Autodesk Inventor part; units mm, degrees
ref_plane "YZ Plane" through (0, 0, 0) normal (1, 0, 0) x (0, 1, 0)
ref_plane "XZ Plane" through (0, 0, 0) normal (0, 1, 0) x (-1, 0, 0)
ref_plane "XY Plane" through (0, 0, 0) normal (0, 0, 1) x (1, 0, 0)
sketch "Boceto1" plane through (0, 0, 0) normal (0, 0, 1) x (1, 0, 0)
  line L0 (567.5, -510) -> (-567.5, -510)
  line L1 (-567.5, -510) -> (-567.5, 510)
  line L2 (-567.5, 510) -> (567.5, 510)
  line L3 (567.5, 510) -> (567.5, -510)
  line L4 (567.5, -510) -> (-567.5, 510) construction
  line L5 (-567.5, -510) -> (567.5, 510) construction
  line L6 (605.6, 548.1) -> (-605.6, 548.1)
  line L7 (-605.6, 548.1) -> (-605.6, -548.1)
  line L8 (-605.6, -548.1) -> (605.6, -548.1)
  line L9 (605.6, -548.1) -> (605.6, 548.1)
  point P0 (0, 0)
  dimension "d0" = 1135
  dimension "d1" = 1020
  dimension "d2" = 38.1
extrude "Extrusión1" add sketch "Boceto1" along normal blind 38.1
fillet "Empalme1" radius 2 8 edges at (605.6, 548.1, 19.05) (605.6, -548.1, 19.05) (-605.6, 548.1, 19.05) (-605.6, -548.1, 19.05) (-567.5, -510, 19.05) (-567.5, 510, 19.05) (567.5, 510, 19.05) (567.5, -510, 19.05)
fillet "Empalme2" radius 2 24 edges at (-605.0142, 547.5142, 38.1) (-605.6, 0, 38.1) (-605.0142, -547.5142, 38.1) (0, -548.1, 38.1) (605.0142, -547.5142, 38.1) (605.6, 0, 38.1) (605.0142, 547.5142, 38.1) (0, 548.1, 38.1) (567.5, 0, 38.1) (0, -510, 38.1) (-567.5, 0, 38.1) (0, 510, 38.1) (-605.0142, 547.5142, 0) (-605.6, 0, 0) (-605.0142, -547.5142, 0) (0, -548.1, 0) (605.0142, -547.5142, 0) (605.6, 0, 0) (605.0142, 547.5142, 0) (0, 548.1, 0) (567.5, 0, 0) (0, -510, 0) (-567.5, 0, 0) (0, 510, 0)
sketch "Boceto2" plane through (0, 0, 0) normal (0, 0, -1) x (-1, 0, 0)
  line L0 (-603.6, 546.1) -> (-603.6, -546.1)
  line L1 (-603.6, 546.1) -> (-543.6, 546.1)
  line L2 (603.6, 546.1) -> (-603.6, 546.1)
  line L3 (-603.6, 548.1) -> (603.6, 548.1)
  line L4 (-543.6, 548.1) -> (-547.6, 548.1)
  line L5 (-543.6, 548.1) -> (-543.6, 544.1)
  line L6 (-543.6, 544.1) -> (-521.6, 544.1)
  line L7 (-521.6, 544.1) -> (-521.6, 548.1)
  line L8 (-521.6, 548.1) -> (-543.6, 548.1)
  line L9 (-543.6, 548.1) -> (-543.6, 544.1)
  line L10 (0, 548.1) -> (0, -512)
  line L11 (565.5, -512) -> (-565.5, -512)
  line L12 (-565.5, 0) -> (567.5, 0)
  line L13 (567.5, -508) -> (567.5, 508)
  line L14 (-603.6, -548.1) -> (603.6, -548.1)
  line L15 (-543.6, -548.1) -> (-543.6, -544.1)
  line L16 (-543.6, -544.1) -> (-521.6, -544.1)
  line L17 (-521.6, -544.1) -> (-521.6, -548.1)
  line L18 (543.6, 548.1) -> (543.6, 544.1)
  line L19 (543.6, 544.1) -> (521.6, 544.1)
  line L20 (521.6, 544.1) -> (521.6, 548.1)
  line L21 (521.6, 548.1) -> (543.6, 548.1)
  line L22 (543.6, -544.1) -> (521.6, -544.1)
  line L23 (521.6, -544.1) -> (521.6, -548.1)
  line L24 (603.6, -548.1) -> (-603.6, -548.1)
  line L25 (543.6, -548.1) -> (543.6, -544.1)
  point P0 (0, 0)
  point P1 (543.6, 546.1)
  dimension "d7" = 60
  dimension "d8" = 4
  dimension "d9" = 4
  dimension "d10" = 22
extrude "Extrusión2" add sketch "Boceto2" along normal blind 40 contours L18 L19 L20 L2 | L2 L20 L3 L18 | L7 L6 L5 L2 | L2 L5 L3 L7 | L15 L16 L17 L14 | L23 L22 L25 L14
fillet "Empalme3" radius 10 8 edges at (543.6, -546.1, -40) (521.6, -546.1, -40) (543.6, 546.1, -40) (521.6, 546.1, -40) (-521.6, 546.1, -40) (-543.6, 546.1, -40) (-543.6, -546.1, -40) (-521.6, -546.1, -40)
sketch "Boceto3" plane through (521.6, -548.1, 0) normal (0, -1, 0) x (1, 0, 0)
  line L0 (22, 0) -> (0, 0)
  line L1 (0, 0) -> (22, 0)
  line L2 (22, 0) -> (22, -40)
  line L3 (22, -40) -> (0, -40)
  line L4 (0, -40) -> (0, 0)
  circle A0 centre (11, -29) radius 11
  circle A1 centre (11, -29) radius 5
  point P0 (-521.6, 0)
  dimension "d14" = 10
extrude "Extrusión3" cut sketch "Boceto3" against normal blind 20000 contours A1
sketch "Boceto4" plane through (-543.6, -548.1, 0) normal (0, -1, 0) x (1, 0, 0)
  line L0 (0, 0) -> (0, -30)
  line L1 (0, 0) -> (22, 0)
  line L2 (22, 0) -> (22, -40)
  line L3 (22, -40) -> (0, -40)
  line L4 (0, -40) -> (0, 0)
  circle A0 centre (11, -29) radius 11
  circle A1 centre (11, -29) radius 5
  point P0 (543.6, 0)
  dimension "d17" = 10
extrude "Extrusión4" cut sketch "Boceto4" against normal blind 20000 contours A1
sketch "Boceto5" plane through (0, 0, 38.1) normal (0, 0, 1) x (1, 0, 0)
  line L0 (-565.5, 510) -> (565.5, 510)
  line L1 (565.5, -510) -> (-565.5, -510)
  point P0 (0, 0)
  dimension "d20" = 1020
sketch "Boceto6" plane through (0, 0, 38.1) normal (0, 0, 1) x (1, 0, 0)
  line L0 (565.5, -510) -> (-565.5, -510)
  line L1 (543.6, -548.1) -> (521.6, -548.1)
  line L2 (565.5, -510) -> (527.4, -510)
  line L3 (527.4, -510) -> (527.4, -548.1)
  line L4 (527.4, -548.1) -> (565.5, -548.1)
  line L5 (565.5, -548.1) -> (565.5, -510)
  line L6 (555.5, -538.1) -> (537.4, -538.1)
  line L7 (537.4, -538.1) -> (537.4, -520)
  line L8 (537.4, -520) -> (555.5, -520)
  line L9 (555.5, -520) -> (555.5, -538.1)
  circle A0 centre (555.5, -538.1) radius 2.5
  circle A1 centre (555.5, -520) radius 2.5
  circle A2 centre (537.4, -538.1) radius 2.5
  circle A3 centre (537.4, -520) radius 2.5
  line L10 (0, 0) -> (0, -570.6664)
  line L11 (0, 0) -> (796.3032, 0)
  line L12 (-565.5, -510) -> (-527.4, -510)
  line L13 (-527.4, -510) -> (-527.4, -548.1)
  line L14 (-527.4, -548.1) -> (-565.5, -548.1)
  line L15 (-565.5, -548.1) -> (-565.5, -510)
  circle A4 centre (-555.5, -538.1) radius 2.5
  circle A5 centre (-555.5, -520) radius 2.5
  circle A6 centre (-537.4, -538.1) radius 2.5
  circle A7 centre (-537.4, -520) radius 2.5
  line L16 (565.5, 510) -> (-565.5, 510)
  line L17 (527.4, 510) -> (527.4, 548.1)
  line L18 (527.4, 548.1) -> (565.5, 548.1)
  line L19 (565.5, 548.1) -> (565.5, 510)
  circle A8 centre (555.5, 538.1) radius 2.5
  circle A9 centre (555.5, 520) radius 2.5
  circle A10 centre (537.4, 538.1) radius 2.5
  circle A11 centre (537.4, 520) radius 2.5
  line L20 (-527.4, 510) -> (-527.4, 548.1)
  line L21 (-527.4, 548.1) -> (-565.5, 548.1)
  line L22 (-565.5, 548.1) -> (-565.5, 510)
  circle A12 centre (-555.5, 538.1) radius 2.5
  circle A13 centre (-537.4, 538.1) radius 2.5
  circle A14 centre (-537.4, 520) radius 2.5
  circle A15 centre (-555.5, 520) radius 2.5
  line L23 (-565.5, 510) -> (-527.4, 510)
  dimension "d21" = 38.1
  dimension "d22" = 10
  dimension "d23" = 5
  dimension "d24" = 5
  dimension "d25" = 5
  dimension "d26" = 5
extrude "Extrusión5" cut sketch "Boceto6" against normal blind 5 contours A2 L7 L6 | L6 L7 A2 | A0 L9 L6 | L6 L9 A0 | A3 L8 L7 | L7 L8 A3 | A1 L8 L9 | L9 L8 A1 | A4 | A5 | A6 | A7 | A8 | A9 | A10 | A11 | A12 | A13 | A14 | A15
equation "\"d27\" = d24"
Here's how the part is built. I have some questions about the finished solid (model axes, mm). A direction names the side the tool comes from. Give positions to 0.01 mm unless a question says otherwise; leave off trailing zeros. Write each loop counter-clockwise with the first axis right and the second up, starting at its lowest first coordinate (ties: lowest second). Pieces come first, ordered by that corner, then holes. Notation, with made-up numbers: (13, 58) -> (61, 58) arc R31 cw to (61, 93) -> close; hole circle Ø8 at (43.25, 13). An arc over 180 degrees is marked (long way). Use one line per item in the form item = value. Start each with the question number.
1. Thinking about a two-plate mould opening in X: for faces 3 (the face through (-8, -548.1, 19)), 4 (the face through (605.6, -8, 19)), 5 (the face through (567.5, 7, 19)), 6 (the face through (-567.5, -7, 19)), which applies, +X half, -X half, draft (parallel to the pull), parting line (faces both ways), or undercut?
2. Will these pins go through, and if not, where does the flat tip stop? pin 1 Ø4 at (x, y) = (555.5, -520) entering from -Z; pin 2 Ø1.5 at (x, y) = (-554.5, 519) entering from +Z; pin 3 Ø2 at (x, y) = (-529, -547.5) entering from +Z.
3. On a 3-axis mill with a long thin cutter (end or side, diameter ignored), from which of +Z, -Z, +X, -X, +Y, -Y can I reach the whole of each face in a straight line? I mean faces 1 (the face through (-605.6, 8, 19)), 2 (the face through (-8, 510, 19)). Say none if no direction works.
4. If I drill on L1, parallel to X at y = 520, z = 35; L2, parallel to Y at x = 537.4, z = 36.55; L3, parallel to Y at x = -375.5, z = 22, over which ranges is the centre line in solid material (lowest first)?
5. Imagine slicing it at B-B on x = -347.5. List the corners of the cut face in (y, z) for me.
6. Imagine slicing it at A-A on y = 26. List the corners of the cut face in (x, z) for me.
Entries:
q1.face_3 = draft
q1.face_4 = +X half
q1.face_5 = undercut
q1.face_6 = undercut
q2.pin_1 = 0
q2.pin_2 = 33.1
q2.pin_3 = 38.06
q3.face_1 = +Z, -Z, -X, +Y, -Y
q3.face_2 = +Z, -Z
q4.L1 = -605.6 to -558, -553 to -539.9, -534.9 to 534.9, 539.9 to 553, 558 to 605.6
q4.L2 = -548.05 to -540.6, -535.6 to -522.5, -517.5 to -510.05, 510.05 to 517.5, 522.5 to 535.6, 540.6 to 548.05
q4.L3 = -548.1 to -510, 510 to 548.1
q5.outline = (-548.1, 2) arc R2 ccw to (-546.1, 0) -> (-512, 0) arc R2 ccw to (-510, 2) -> (-510, 36.1) arc R2 ccw to (-512, 38.1) -> (-546.1, 38.1) arc R2 ccw to (-548.1, 36.1) -> close; (510, 2) arc R2 ccw to (512, 0) -> (546.1, 0) arc R2 ccw to (548.1, 2) -> (548.1, 36.1) arc R2 ccw to (546.1, 38.1) -> (512, 38.1) arc R2 ccw to (510, 36.1) -> close
q6.outline = (-605.6, 2) arc R2 ccw to (-603.6, 0) -> (-569.5, 0) arc R2 ccw to (-567.5, 2) -> (-567.5, 36.1) arc R2 ccw to (-569.5, 38.1) -> (-603.6, 38.1) arc R2 ccw to (-605.6, 36.1) -> close; (567.5, 2) arc R2 ccw to (569.5, 0) -> (603.6, 0) arc R2 ccw to (605.6, 2) -> (605.6, 36.1) arc R2 ccw to (603.6, 38.1) -> (569.5, 38.1) arc R2 ccw to (567.5, 36.1) -> close
